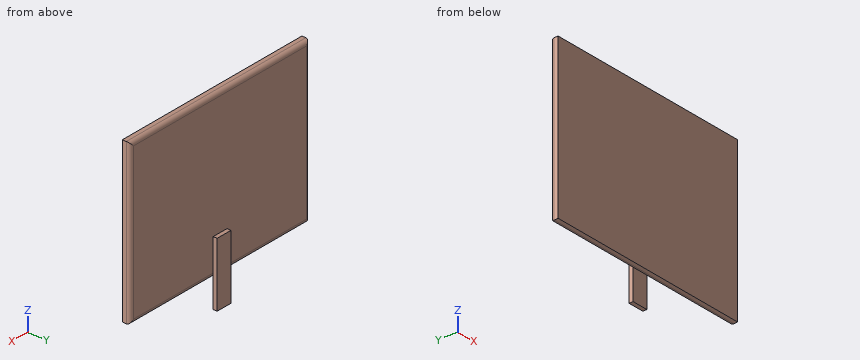
```python
from build123d import *

# Parameters (mm, degrees)
F0_W     = 660.4
F0_H     = 508
F1_DEPTH = 25.4
F2_R     = 12.7
F3_W     = 50.8
F3_H     = 203.2
F4_DEPTH = 12.7


with BuildPart() as f1:
    # F0 (on Front) → F1 (new body)
    with BuildSketch(Plane.XZ):
        with Locations((330.2, 254)):
            Rectangle(F0_W, F0_H)
    extrude(amount=F1_DEPTH)

    # F2
    f2_edges = [f1.edges().sort_by_distance(p)[0] for p in [
        (330.2, 0, 508),
        (660.4, 0, 254),
        (330.2, 0, 0),
        (0, 0, 254),
    ]]
    fillet(f2_edges, radius=F2_R)

    # F3 (on face) → F4 (join)
    with BuildSketch(Plane(origin=(0, 0, 0), x_dir=(-1, 0, 0), z_dir=(0, 1, 0))):
        with Locations((-330.2, 12.7)):
            Rectangle(F3_W, F3_H)
    extrude(amount=F4_DEPTH)


solid = f1.part
```
Read the model definition and answer for the solid it produces. Units are mm, in the model's axes. Give positions to 0.01 mm unless a question says otherwise; leave off trailing zeros. Loops run counter-clockwise (first coordinate to the right, second up) from the corner with the lowest first, then second, coordinate; pieces in that order, holes last.
Item 1: The part is cut by section D-D (x = 205.5). Write down the section's boundary in (y, z).
Item 2: Each of these flat-tipped pins is pushed along its axis until it touches: pin 1 Ø3 at (y, z) = (0.5, 137) entering from -X; pin 2 Ø6 at (x, z) = (376, 320.5) entering from +Y; pin 3 Ø1 at (x, y) = (553, -20.5) entering from -Z. Where does it stop, or does it pass through?
Item 3: The part is cut by section C-C (z = 303). Write down the section's boundary in (x, y).
Item 4: Find the intervals of material crossed by line 1 along Y through (x, z) = (517, 26); line 2 along Z through (x, y) = (430, -23); line 3 along X through (y, z) = (3, 1.5), in increasing order.
Item 5: The part is cut by section B-B (z = 28.5). Write down the section's boundary in (x, y).
Item 6: The part is cut by section A-A (x = 342). Write down the section's boundary in (y, z), and give its area (3 significant figures).
Taken from the geometry:
1. outline: (-25.4, 0) - (-12.7, 0) arc R12.7 ccw to (0, 12.7) - (0, 495.3) arc R12.7 ccw to (-12.7, 508) - (-25.4, 508) - close
2. pin 1: stops at x = 7.76
2. pin 2: stops at y = 0
2. pin 3: stops at z = 0
3. outline: (0, -25.4) - (660.4, -25.4) - (660.4, -12.7) arc R12.7 ccw to (647.7, 0) - (12.7, 0) arc R12.7 ccw to (0, -12.7) - close
4. line 1: y = -25.4 to 0
4. line 2: z = 0 to 508
4. line 3: x = 304.8 to 355.6
5. outline: (0, -25.4) - (660.4, -25.4) - (660.4, -12.7) arc R12.7 ccw to (647.7, 0) - (355.6, 0) - (355.6, 12.7) - (304.8, 12.7) - (304.8, 0) - (12.7, 0) arc R12.7 ccw to (0, -12.7) - close
6. outline: (-25.4, 0) - (-12.7, 0) arc R12.7 ccw to (0, 12.7) - (0, -88.9) - (12.7, -88.9) - (12.7, 114.3) - (0, 114.3) - (0, 495.3) arc R12.7 ccw to (-12.7, 508) - (-25.4, 508) - close
6. area: 15,400 mm2
